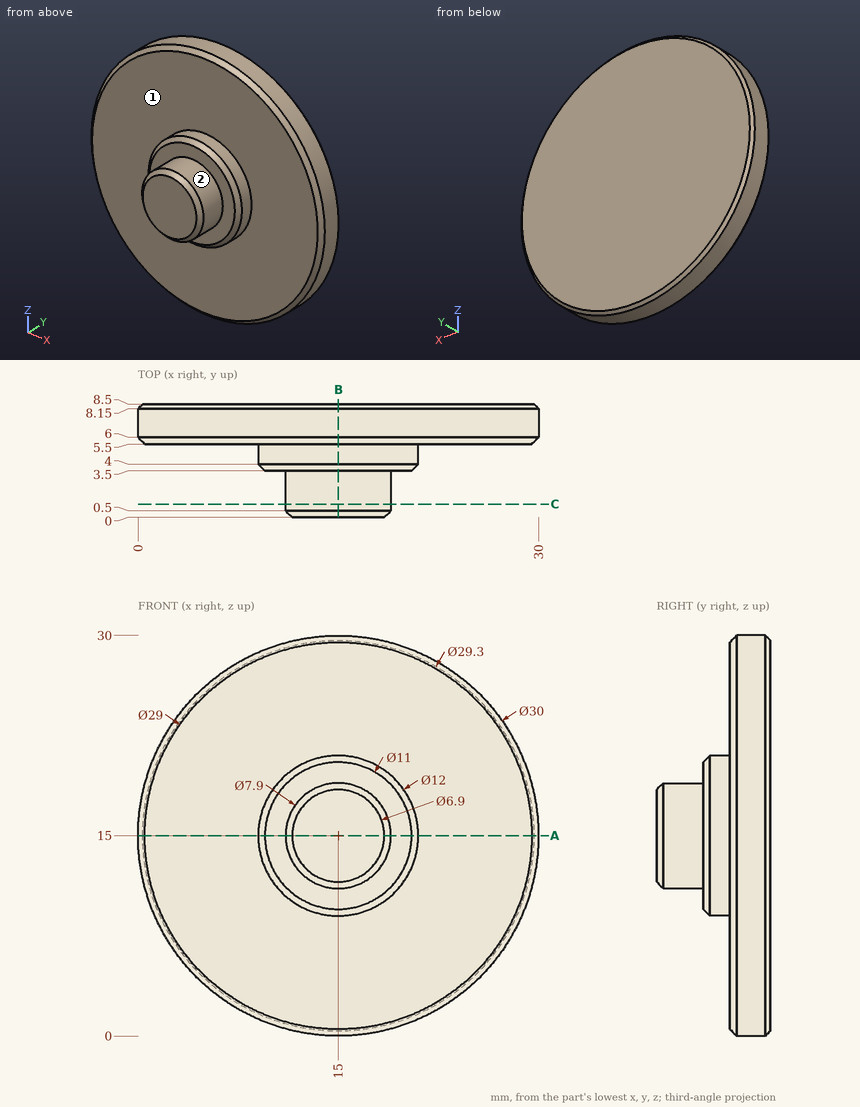
Here's the drawing with two shaded views (mm, measured from the low corner). I have some questions. Give positions to 0.01 mm unless a question says otherwise; leave off trailing zeros. Order: outer loops, then holes, each group sorted by start corner. A loop starts at its lowest first (then second) coordinate and runs counter-clockwise, first axis right, second up. Notation, with made-up numbers: (72.5, -3.5) -> (100.5, -3.5) arc R4 ccw to (100.5, 1.5) -> close; hole circle Ø7 at (-5, 18). An arc over 180 degrees is marked (long way). Use a Markdown table: item, result. Add a question column.
Item 1: Imagine slicing it at C-C on y = 1. Please give me the cut outline in (x, z), plus the area to 3 significant figures.
Item 2: Will these pins go through, and if not, where does the flat tip stop? pin 1 (1.5 mm diameter, centred on x = 23.5, y = 5, fed in from +Z); pin 2 (1 mm diameter, centred on x = 19, z = 21.5, fed in from -Y); pin 3 (4 mm diameter, centred on x = 21, y = 4, fed in from +Z).
Item 3: I need wall thicknesses on line 1 (Y direction, x = 21.5, z = 12); line 2 (Y direction, x = 12, z = 10.5); line 3 (Z direction, x = 25.75, y = 8.25). Which ranges of each line are inside material? Lowest first, please.
Item 4: Imagine slicing it at B-B on x = 15. Please give me the cut outline in (y, z).
Item 5: Imagine slicing it at A-A on z = 15. Please give me the cut outline in (x, y).
Item 6: If we mould it in two halves opening along X, with no side actions, what happens to the marked faces 1 and 2? For each: pulls with the +X half, pulls with the -X half, needs draft (parallel to the pull), parting line crosses it, or undercut.
Data:
| question | item | result |
|---|---|---|
| 1 | outline | circle Ø7.9 at (15, 15) |
| 1 | area | 49.0 mm² |
| 2 | pin 1 | stops at z = 27.19 |
| 2 | pin 2 | stops at y = 5.5 |
| 2 | pin 3 | stops at z = 28.9 |
| 3 | line 1 | y = 5.5 to 8.5 |
| 3 | line 2 | y = 3.5 to 8.5 |
| 3 | line 3 | z = 4.68 to 25.32 |
| 4 | outline | (0, 11.55) -> (0.5, 11.05) -> (3.5, 11.05) -> (3.5, 9.5) -> (4, 9) -> (5.5, 9) -> (5.5, 0.5) -> (6, 0) -> (8.15, 0) -> (8.5, 0.35) -> (8.5, 29.65) -> (8.15, 30) -> (6, 30) -> (5.5, 29.5) -> (5.5, 21) -> (4, 21) -> (3.5, 20.5) -> (3.5, 18.95) -> (0.5, 18.95) -> (0, 18.45) -> close |
| 5 | outline | (0, 6) -> (0.5, 5.5) -> (9, 5.5) -> (9, 4) -> (9.5, 3.5) -> (11.05, 3.5) -> (11.05, 0.5) -> (11.55, 0) -> (18.45, 0) -> (18.95, 0.5) -> (18.95, 3.5) -> (20.5, 3.5) -> (21, 4) -> (21, 5.5) -> (29.5, 5.5) -> (30, 6) -> (30, 8.15) -> (29.65, 8.5) -> (0.35, 8.5) -> (0, 8.15) -> close |
| 6 | face 1 | needs draft |
| 6 | face 2 | parting line crosses it |
